```python
from build123d import *

# Parameters (mm, degrees)
F0_W        = 45
F0_H        = 45
F1_DEPTH    = 33
F3_DEPTH    = 55.8
F4_R        = 6.5
F5_DEPTH    = 68.3
F6_T1_DEPTH = 57.1976554231
F6_T3_DEPTH = 62.61396425
F6_T5_DEPTH = 70.7168298797
F7_R        = 5


# Not quite as in the source:
# - a fillet or chamfer that OpenCascade refuses, or shapes differently, is made with other operations: its cross-section is extruded or revolved along the edge and cut away or added


with BuildPart() as f1:
    # F0 (on Front) → F1 (new body)
    with BuildSketch(Plane.XZ):
        Rectangle(F0_W, F0_H)
    extrude(amount=F1_DEPTH)

    # F2 (on face) → F3 (cut)
    with BuildSketch(Plane.XY.offset(22.5)):
        Polygon((22.5, -33), (22.5, 0), (8.9808255434, -33), align=None)
    extrude(amount=-F3_DEPTH, mode=Mode.SUBTRACT)

    # F4 (on face) → F5 (cut)
    with BuildSketch(Plane.XZ.offset(33)):
        with Locations((-8.7795946747, 0)):
            Circle(F4_R)
    extrude(amount=-F5_DEPTH, mode=Mode.SUBTRACT)

    # F6: chamfer of 5 on 4 edges, made by hand

    # F6_s2 → F6_t1 (cut)
    with BuildSketch(Plane.YZ.offset(-35.3584149398)):
        Polygon((-28, 22.5), (-33, 17.5), (-33, 22.5), align=None)
        Polygon((-28, -22.5), (-33, -17.5), (-33, -22.5), align=None)
    extrude(amount=F6_T1_DEPTH, mode=Mode.SUBTRACT)

    # F6_s4 → F6_t3 (cut)
    with BuildSketch(Plane.XY.offset(-31.306982125)):
        Polygon((10.252665661, -29.8954669522), (5.6258735721, -33), (8.9808255434, -33), align=None)
    extrude(amount=F6_T3_DEPTH, mode=Mode.SUBTRACT)

    # F6_s6 → F6_t5 (cut)
    with BuildSketch(Plane.XY.offset(-35.3584149398)):
        Polygon((-22.5, -28), (-17.5, -33), (-22.5, -33), align=None)
    extrude(amount=F6_T5_DEPTH, mode=Mode.SUBTRACT)

    # F7
    f7_edges = [f1.edges().sort_by_distance(p)[0] for p in [
        (-5.937063, -33, 17.5),
        (5.625874, -33, 0),
        (-5.937063, -33, -17.5),
        (-17.5, -33, 0),
    ]]
    fillet(f7_edges, radius=F7_R)


solid = f1.part
```
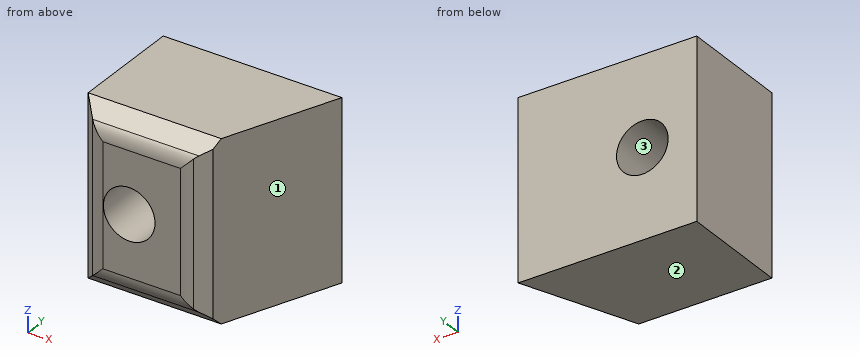
The model under review builds one solid part; all positions refer to its coordinate system, in mm. Face numbers are marked on the shaded views. Round coordinates to 2 decimals unless told otherwise and drop trailing zeros. Write each loop counter-clockwise with the first axis right and the second up, starting at its lowest first coordinate (ties: lowest second). Pieces come first, ordered by that corner, then holes. Notation, with made-up numbers: (87, 53) - (106, 53) arc R32 cw to (106, 84) - close; hole circle Ø3 at (-38, 48). An arc over 180 degrees is marked (long way). One line per question, with ' | ' between items.
Item 1: To check wall thickness, follow probe 1 along X at (y, z) = (-23, 3); probe 2 along Z at (x, y) = (-3.5, -22); probe 3 along X at (y, z) = (-3, 5). State the ranges of each line that lie inside material, in increasing order.
Resolved:
probe 1: x = -22.5 to -14.55, -3.01 to 13.08 | probe 2: z = -22.5 to -3.79, 3.79 to 22.5 | probe 3: x = -22.5 to -12.93, -4.63 to 21.27
Item 2: Add section A-A, the plane z = 0. Give the boundary of the cut face in (x, y).
Resolved:
outline: (-22.5, -28) - (-18.96, -31.54) arc R5 ccw to (-15.43, -33) - (-15.28, -33) - (-15.28, 0) - (-22.5, 0) - close; (-2.28, -33) - (4.1, -33) arc R5 ccw to (6.89, -32.15) - (10.25, -29.9) - (22.5, 0) - (-2.28, 0) - close
Item 3: Add section C-C, the plane z = 11. Give the boundary of the cut face in (x, y), then the cut area to 3 significant figures.
Resolved:
outline: (-22.5, -28) - (-18.96, -31.54) arc R5 ccw to (-15.43, -33) - (4.1, -33) arc R5 ccw to (6.89, -32.15) - (10.25, -29.9) - (22.5, 0) - (-22.5, 0) - close | area: 1,240 mm2
Item 4: Add section D-D, the plane y = -24. Give the boundary of the cut face in (x, z), then the cut area to 3 significant figures.
Resolved:
outline: (-22.5, -22.5) - (12.67, -22.5) - (12.67, 22.5) - (-22.5, 22.5) - close; hole circle Ø13 at (-8.78, 0) | area: 1,450 mm2
Item 5: The part is to be moulded in two halves that separate along Z. For the marked faces 1, 2 and 3, say which applies: pulls with the +Z half, pulls with the -Z half, needs draft (parallel to the pull), parting line crosses it, or undercut.
Resolved:
face 1: needs draft | face 2: pulls with the -Z half | face 3: undercut
Item 6: Add section B-B, the plane x = -1. Give the boundary of the cut face in (y, z).
Resolved:
outline: (-33, -15.43) arc R5 ccw to (-31.54, -18.96) - (-28, -22.5) - (0, -22.5) - (0, 22.5) - (-28, 22.5) - (-31.54, 18.96) arc R5 ccw to (-33, 15.43) - close
Item 7: For P1, Ø4, axis at y = -11, z = 14, coming from the +X side; P2, Ø8, axis at x = -8.78, z = 0, coming from the +Y side; P3, Ø10, axis at y = -17.5, z = -6.5, coming from the +X side, all flat-tipped, find the tip position at first contact; note any pin that passes through.
Resolved:
P1: stops at x = 18.81 | P2: passes through | P3: stops at x = 17.38
